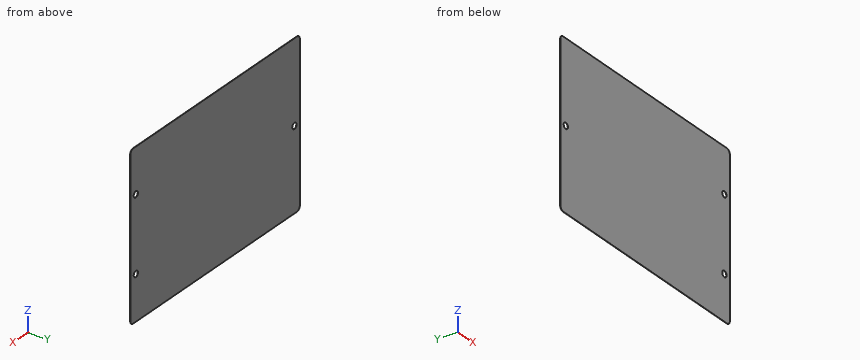
```python
from build123d import *

# Parameters (mm, degrees)
SKETCH1_W           = 189
SKETCH1_H           = 132
SKETCH1_R           = 2.4
BOSS_EXTRUDE1_DEPTH = 0.2
FILLET1_R           = 3


with BuildPart() as part:
    # Sketch1 → Boss-Extrude1 (new body)
    with BuildSketch(Plane(origin=(0, 0, 0), x_dir=(1, 0, 0), z_dir=(0, 1, 0))):
        with Locations((94.5, 66)):
            Rectangle(SKETCH1_W, SKETCH1_H)
        with Locations(Location((6, 66, 0), (0, 0, 270))):
            Circle(SKETCH1_R, mode=Mode.SUBTRACT)
        with Locations(Location((183, 36, 0), (0, 0, 270))):
            Circle(SKETCH1_R, mode=Mode.SUBTRACT)
        with Locations(Location((183, 96, 0), (0, 0, 270))):
            Circle(SKETCH1_R, mode=Mode.SUBTRACT)
    extrude(amount=BOSS_EXTRUDE1_DEPTH)

    # Fillet1
    fillet1_edges = [part.edges().sort_by_distance(p)[0] for p in [
        (0, 0.1, -132),
        (189, 0.1, -132),
        (189, 0.1, 0),
        (0, 0.1, 0),
    ]]
    fillet(fillet1_edges, radius=FILLET1_R)


solid = part.part
```
The listing builds one solid part. Answer for the finished solid, in the listing's coordinates (mm). Give positions to 0.01 mm unless a question says otherwise; leave off trailing zeros. Loops run counter-clockwise (first coordinate to the right, second up) from the corner with the lowest first, then second, coordinate; pieces in that order, holes last. Notation, with made-up numbers: (63, 38.5) - (120, 38.5) arc R11 ccw to (120, 53.5) - close; hole circle Ø11 at (-15, 30.5). An arc over 180 degrees is marked (long way). Return JSON: item names as keys, results as strings. Group by question number.
1. Given pin 1 Ø4 at (x, z) = (183, -96) entering from -Y, flat-ended and moving along its own axis, determine where the tip first touches the part or whether it passes through.
2. Find section A-A (x = 183). Write down the section's boundary in (y, z), then the cut area to 3 significant figures.
3. Find section B-B (z = -96). Write down the section's boundary in (x, y).
4. Straight lines are drawn through the part: line 1 (Z direction, x = 183, y = 0.1); line 2 (X direction, y = 0.15, z = -96); line 3 (X direction, y = 0.1, z = -35). For each, find the intervals that lie inside material, in ascending order. Write a range as [from, to].
5. Find section C-C (x = 6). Write down the section's boundary in (y, z), then the cut area to 3 significant figures.
Verdict:
{
 "1": {"pin 1": "passes through"},
 "2": {"outline": "(0, -132) - (0.2, -132) - (0.2, -98.4) - (0, -98.4) - close; (0, -93.6) - (0.2, -93.6) - (0.2, -38.4) - (0, -38.4) - close; (0, -33.6) - (0.2, -33.6) - (0.2, 0) - (0, 0) - close", "area": "24.5 mm^2"},
 "3": {"outline": "(0, 0) - (180.6, 0) - (180.6, 0.2) - (0, 0.2) - close; (185.4, 0) - (189, 0) - (189, 0.2) - (185.4, 0.2) - close"},
 "4": {"line 1": "z = [-132, -98.4], [-93.6, -38.4], [-33.6, 0]", "line 2": "x = [0, 180.6], [185.4, 189]", "line 3": "x = [0, 180.82], [185.18, 189]"},
 "5": {"outline": "(0, -132) - (0.2, -132) - (0.2, -68.4) - (0, -68.4) - close; (0, -63.6) - (0.2, -63.6) - (0.2, 0) - (0, 0) - close", "area": "25.4 mm^2"}
}
